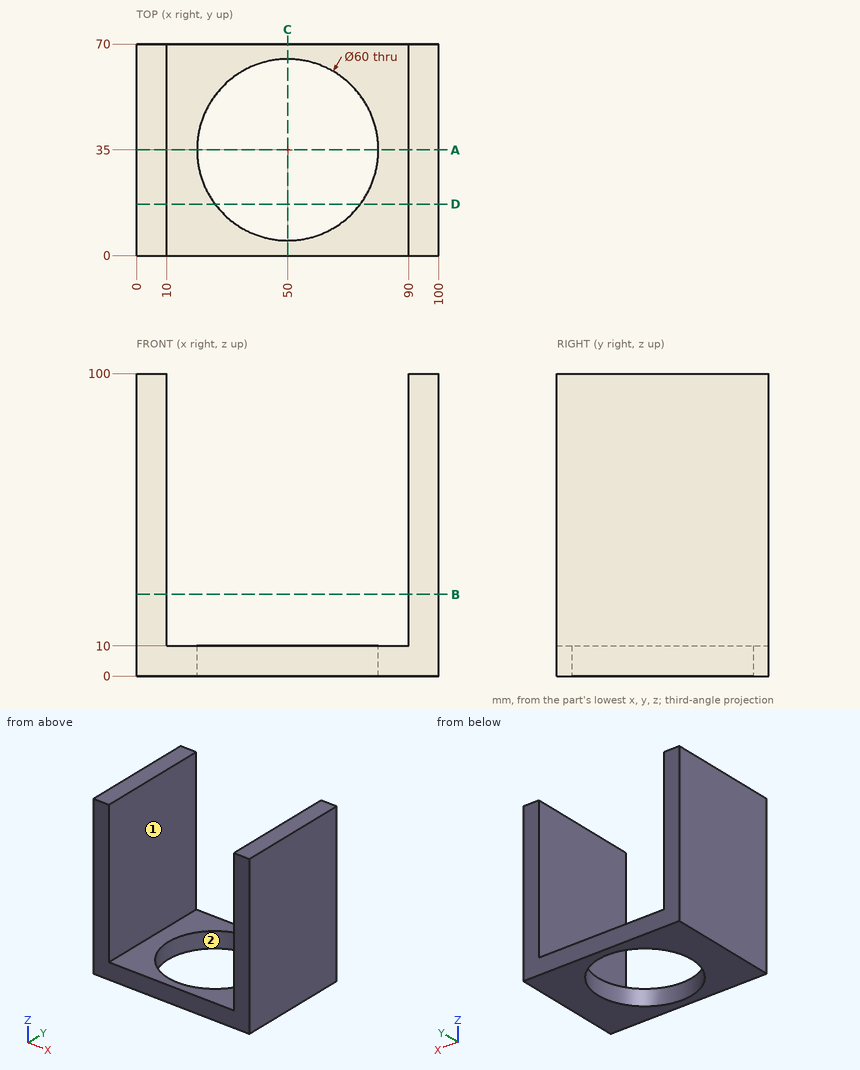
Design review of the part shown in the three views and the two pictorial views. Dimensions are in mm from the part's minimum x, y and z. A direction names the side the tool comes from. Round coordinates to 2 decimals unless told otherwise and drop trailing zeros. Order: outer loops, then holes, each group sorted by start corner. A loop starts at its lowest first (then second) coordinate and runs counter-clockwise, first axis right, second up. Notation, with made-up numbers: M 47,69.5 L 53,69.5 A22 cw 53,101.5 Z; hole C 12.5,5.5 d2. An arc over 180 degrees is marked long. Put each result on its own line as item: value.
Q1. Consider section C-C (x = 50). State the section outline as (y, z) points.
Reported:
outline: M 0,0 L 5,0 L 5,10 L 0,10 Z; M 65,0 L 70,0 L 70,10 L 65,10 Z
Q2. Consider section D-D (y = 17). State the section outline as (x, z) points.
Reported:
outline: M 0,0 L 26,0 L 26,10 L 10,10 L 10,100 L 0,100 Z; M 74,0 L 100,0 L 100,100 L 90,100 L 90,10 L 74,10 Z
Q3. To check wall thickness, follow line 1 (X direction, y = 65, z = 50.5); line 2 (Y direction, x = 50, z = 6); line 3 (Z direction, x = 26, y = 12). State the ranges of each line that lie inside material, in increasing order.
Reported:
line 1: 0 to 10, 90 to 100
line 2: 0 to 5, 65 to 70
line 3: 0 to 10
Q4. Machinability: for the marked faces 1 and 2, which of the approach directions +Z, -Z, +X, -X, +Y, -Y give a long, thin tool a straight path to every point of the face, cutting with its end or side? Answer none if there is none.
Reported:
face 1: +Z, +Y, -Y
face 2: +Z, -Z
Q5. Insertion check: pin 1 Ø1 at (y, z) = (35, 44.5) entering from -X; pin 2 Ø1.5 at (x, y) = (82, 13) entering from +Z. Each pin has a flat end and moves straight along its axis. Give the tip position at first contact, or say it passes through.
Reported:
pin 1: x = 0
pin 2: z = 10
Q6. Consider section A-A (y = 35). State the section outline as (x, z) points.
Reported:
outline: M 0,0 L 20,0 L 20,10 L 10,10 L 10,100 L 0,100 Z; M 80,0 L 100,0 L 100,100 L 90,100 L 90,10 L 80,10 Z
Q7. Consider section B-B (z = 27). State the section outline as (x, y) points, and give its area (3 significant figures).
Reported:
outline: M 0,0 L 10,0 L 10,70 L 0,70 Z; M 90,0 L 100,0 L 100,70 L 90,70 Z
area: 1,400 mm²
